from build123d import *

# Parameters (mm, degrees)
SKETCH1_W               = 98.425
SKETCH1_H               = 91.28125
SKETCH1_R               = 5.159375
BOSS_EXTRUDE1_DEPTH     = 3.175
SKETCH2_W               = 25.4
SKETCH2_H               = 133.35
BOSS_EXTRUDE3_DEPTH     = 3.175
SKETCH3_W               = 25.4
SKETCH3_H               = 3.175
BOSS_EXTRUDE4_DEPTH     = 38.1
SKETCH4_R               = 4.7625
CUT_EXTRUDE1_DEPTH      = 134.35
SKETCH5_R               = 5.159375
BOSS_EXTRUDE5_DEPTH     = 9.525
SKETCH6_R               = 6.35
BOSS_EXTRUDE6_DEPTH     = 4.7625
SKETCH7_W               = 98.425
SKETCH7_H               = 3.175
BOSS_EXTRUDE7_DEPTH     = 69.85
CUT_EXTRUDE2_DEPTH      = 16.875
CUT_EXTRUDE2_DEPTH_BACK = 118.475


with BuildPart() as part:
    # Sketch1 → Boss-Extrude1 (new body)
    with BuildSketch(Plane(origin=(0, 0, 0), x_dir=(1, 0, 0), z_dir=(0, 1, 0))):
        with Locations((49.2125, 45.640625)):
            Rectangle(SKETCH1_W, SKETCH1_H)
        with Locations((17.065625, 45.640625)):
            Circle(SKETCH1_R, mode=Mode.SUBTRACT)
        with BuildLine():
            Line((11.90625, 66.278125), (11.90625, 75.803125))
            ThreePointArc((11.90625, 75.803125), (17.065625, 80.9625), (22.225, 75.803125))
            Line((22.225, 75.803125), (22.225, 66.278125))
            ThreePointArc((22.225, 66.278125), (17.065625, 61.11875), (11.90625, 66.278125))
        make_face(mode=Mode.SUBTRACT)
        with BuildLine():
            Line((11.90625, 25.003125), (11.90625, 15.478125))
            ThreePointArc((11.90625, 15.478125), (17.065625, 10.31875), (22.225, 15.478125))
            Line((22.225, 15.478125), (22.225, 25.003125))
            ThreePointArc((22.225, 25.003125), (17.065625, 30.1625), (11.90625, 25.003125))
        make_face(mode=Mode.SUBTRACT)
        with BuildLine():
            Line((80.565625, 50.8), (90.090625, 50.8))
            ThreePointArc((90.090625, 50.8), (95.25, 45.640625), (90.090625, 40.48125))
            Line((90.090625, 40.48125), (80.565625, 40.48125))
            ThreePointArc((80.565625, 40.48125), (75.40625, 45.640625), (80.565625, 50.8))
        make_face(mode=Mode.SUBTRACT)
    extrude(amount=BOSS_EXTRUDE1_DEPTH)

    # Sketch2 → Boss-Extrude3 (add)
    with BuildSketch(Plane.XZ):
        with Locations((17.065625, -50.8)):
            Rectangle(SKETCH2_W, SKETCH2_H)
        with Locations((85.725, -50.8)):
            Rectangle(SKETCH2_W, SKETCH2_H)
    extrude(amount=BOSS_EXTRUDE3_DEPTH)

    # Sketch3 → Boss-Extrude4 (add)
    with BuildSketch(Plane.XZ.offset(3.175)):
        with Locations((17.065625, 14.2875)):
            Rectangle(SKETCH3_W, SKETCH3_H)
        with Locations((17.065625, -115.8875)):
            Rectangle(SKETCH3_W, SKETCH3_H)
        with Locations((85.725, 14.2875)):
            Rectangle(SKETCH3_W, SKETCH3_H)
        with Locations((85.725, -115.8875)):
            Rectangle(SKETCH3_W, SKETCH3_H)
    extrude(amount=BOSS_EXTRUDE4_DEPTH)

    # Sketch4 → Cut-Extrude1 (cut, through all)
    with BuildSketch(Plane.XY.offset(15.875)):
        with Locations((15.95994836, -22.225)):
            Circle(SKETCH4_R)
        with Locations((85.725, -22.225)):
            Circle(SKETCH4_R)
    extrude(amount=-CUT_EXTRUDE1_DEPTH, mode=Mode.SUBTRACT)

    # Sketch5 → Boss-Extrude5 (add)
    with BuildSketch(Plane(origin=(0, 3.175, 0), x_dir=(1, 0, 0), z_dir=(0, 1, 0))):
        with Locations((17.065625, 45.640625)):
            Circle(SKETCH5_R)
        with Locations((17.065625, 66.278125)):
            Circle(SKETCH5_R)
        with Locations((90.090625, 45.640625)):
            Circle(SKETCH5_R)
    extrude(amount=-BOSS_EXTRUDE5_DEPTH)

    # Sketch6 → Boss-Extrude6 (add)
    with BuildSketch(Plane(origin=(0, 3.175, 0), x_dir=(1, 0, 0), z_dir=(0, 1, 0))):
        with Locations((90.090625, 45.640625)):
            Circle(SKETCH6_R)
        with Locations((17.065625, 45.640625)):
            Circle(SKETCH6_R)
        with Locations((17.065625, 66.278125)):
            Circle(SKETCH6_R)
    extrude(amount=BOSS_EXTRUDE6_DEPTH)

    # Sketch7 → Boss-Extrude7 (add)
    with BuildSketch(Plane(origin=(0, 3.175, 0), x_dir=(1, 0, 0), z_dir=(0, 1, 0))):
        with Locations((49.2125, 89.69375)):
            Rectangle(SKETCH7_W, SKETCH7_H)
        with Locations((49.2125, 1.5875)):
            Rectangle(SKETCH7_W, SKETCH7_H)
    extrude(amount=BOSS_EXTRUDE7_DEPTH)

    # Sketch8 → Cut-Extrude2 (cut, two sides)
    with BuildSketch(Plane.XY) as cut_extrude2_sk:
        with BuildLine():
            Line((79.375, 73.025), (98.425, 73.025))
            Line((98.425, 73.025), (98.425, 53.975))
            ThreePointArc((98.425, 53.975), (92.845384182, 67.445384182), (79.375, 73.025))
        make_face()
        with BuildLine():
            Line((19.05, 73.025), (0, 73.025))
            Line((0, 73.025), (0, 53.975))
            ThreePointArc((0, 53.975), (5.579615818, 67.445384182), (19.05, 73.025))
        make_face()
    extrude(amount=CUT_EXTRUDE2_DEPTH, mode=Mode.SUBTRACT)
    extrude(cut_extrude2_sk.sketch, amount=-CUT_EXTRUDE2_DEPTH_BACK, mode=Mode.SUBTRACT)


solid = part.part
CAD build for the part. Positions are in the model's coordinates, mm. A direction names the side the tool comes from. Coordinates: 2 decimals unless noted, no trailing zeros. Loops run counter-clockwise (first coordinate to the right, second up) from the corner with the lowest first, then second, coordinate; pieces in that order, holes last. Notation, with made-up numbers: (1.5, -23) - (10.5, -23) arc R22 ccw to (10.5, 15) - close; hole circle Ø9 at (39, 39). An arc over 180 degrees is marked (long way). Write item = value, one per line. Start each with the question number.
Q1. Cut at C-C, the plane x = 63. List the corners of the cut face in (y, z) (3 decimals), then the cut area to 3 significant figures.
Q2. Drill centre lines: L1, parallel to Z at x = 7, y = -18 (3 decimals); L2, parallel to Z at x = 68.5, y = 39 (3 decimals); L3, parallel to Y at x = 17.5, z = -3.5 (3 decimals). Where is each one in solid material? Low to high.
Q3. Which spindle directions (+Z, -Z, +X, -X, +Y, -Y) get a long thin tool onto all of the face, cutting with end or side? Do faces 4 (the flat face through (49, 38, -3.175)), 5 (the flat face through (51, 0, -46)), 6 (the flat face through (83, -18, -114.3)), 7 (the flat face through (17, 0, -104)). Say none if no direction does.
Q4. Cut at B-B, the plane z = -95.5. List the corners of the cut face in (x, y) (3 decimals).
Q5. Cut at A-A, the plane y = -31. List the corners of the cut face in (x, z) (3 decimals), then the cut area to 3 significant figures.
Q6. Flat gauge pins, fed straight in: pin 1 Ø5 at (x, z) = (37, -36) entering from +Y (3 decimals); pin 2 Ø5 at (x, z) = (19.5, 11.5) entering from +Y; pin 3 Ø1 at (x, y) = (68.5, 39.5) entering from -Z; pin 4 Ø20.5 at (y, z) = (-18.5, -77.5) entering from +X. Where does each tip first touch, or does it go through?
Q7. Cut at D-D, the plane y = 61. List the corners of the cut face in (x, z) (3 decimals).
Q8. Pull direction Y, two halves, no side cores. Call faces 1 (the flat face through (73.025, -2, -56)), 2 (the flat face through (49, 73.025, -90)), 3 (the cylindrical face through (84.932, 1.61, -45.754)): pulls with the +Y half, pulls with the -Y half, needs draft (parallel to the pull), parting line crosses it, or undercut.
Computed:
q1.outline = (0, -91.281) - (73.025, -91.281) - (73.025, -88.106) - (3.175, -88.106) - (3.175, -3.175) - (73.025, -3.175) - (73.025, 0) - (0, 0) - close
q1.area = 733 mm²
q2.L1 = -117.475 to -114.3, 12.7 to 15.875
q2.L2 = -91.281 to -88.106, -3.175 to 0
q2.L3 = -3.175 to 3.175
q3.face_4 = +X, -X, +Y
q3.face_5 = +Z, -Z, -Y
q3.face_6 = +X, -X, -Y
q3.face_7 = -Z, +X, -X, +Y
q4.outline = (4.366, -3.175) - (29.766, -3.175) - (29.766, 0) - (4.366, 0) - close; (73.025, -3.175) - (98.425, -3.175) - (98.425, 0) - (73.025, 0) - close
q5.outline = (4.366, -117.475) - (29.766, -117.475) - (29.766, -114.3) - (4.366, -114.3) - close; (4.366, 12.7) - (29.766, 12.7) - (29.766, 15.875) - (4.366, 15.875) - close; (73.025, -117.475) - (98.425, -117.475) - (98.425, -114.3) - (73.025, -114.3) - close; (73.025, 12.7) - (98.425, 12.7) - (98.425, 15.875) - (73.025, 15.875) - close
q5.area = 323 mm²
q6.pin_1 = 3.175
q6.pin_2 = 0
q6.pin_3 = -91.28
q6.pin_4 = through
q7.outline = (1.343, -91.281) - (97.082, -91.281) - (97.082, -88.106) - (1.343, -88.106) - close; (1.343, -3.175) - (97.082, -3.175) - (97.082, 0) - (1.343, 0) - close
q8.face_1 = needs draft
q8.face_2 = pulls with the +Y half
q8.face_3 = undercut
